```python
from build123d import *

# Parameters (mm, degrees)
F0_W     = 206
F0_H     = 56
F1_DEPTH = 3
F2_W     = 206
F2_H     = 56
F3_DEPTH = 10


with BuildPart() as f1:
    # F0 (on Top) → F1 (new body)
    with BuildSketch(Plane.XY):
        Rectangle(F0_W, F0_H)
    extrude(amount=F1_DEPTH)

    # F2 (on face) → F3 (join)
    with BuildSketch(Plane.XY.offset(3)):
        Rectangle(F2_W, F2_H)
        Polygon((100, -25), (-100, -25), (-100, 8.5), (100, -11.5), align=None, mode=Mode.SUBTRACT)
        Polygon((-100, 11.5), (-100, 25), (100, 25), (100, -8.5), align=None, mode=Mode.SUBTRACT)
    extrude(amount=F3_DEPTH)


solid = f1.part
```
Part model, mm, in its own coordinate system. A direction names the side the tool comes from. Round coordinates to 2 decimals unless told otherwise and drop trailing zeros. Loops run counter-clockwise (first coordinate to the right, second up) from the corner with the lowest first, then second, coordinate; pieces in that order, holes last.
Item 1: 3-axis set-ups, long thin cutter, end or side, ignore diameter. For faces 5 (the face through (103, 0, 6)), 6 (the face through (21, 12, 3)): which of +Z, -Z, +X, -X, +Y, -Y reach the whole face in a straight line?
Item 2: Drop a flat-ended pin along its axis: P1, Ø8, axis at x = -69.5, y = 13, coming from the +Z side. Give the stop position or say it passes through.
Item 3: Mould opens along Y. For faces 1 (the face through (1.4, 1.36, 7.93)), 2 (the face through (-1, -28, 6)), 3 (the face through (-1, 28, 6)), 4 (the face through (-8, 0, 13)) say: +Y half, -Y half, draft (parallel to the pull), parting line (faces both ways), or undercut.
Item 4: Drill centre lines: line 1 (X direction, y = -12, z = 10); line 2 (Y direction, x = 49, z = 4.25); line 3 (Y direction, x = -85, z = 8.5). Where is each one in solid material? Low to high.
Item 5: Cut at D-D, the plane y = 1. Give the cut face in (x, z).
Item 6: Cut at C-C, the plane y = -18. Give the cut face in (x, z), then the cut area to 3 significant figures.
Item 7: Cut at B-B, the plane x = -43. Give the cut face in (y, z), then the cut area to 3 significant figures.
Item 8: Cut at A-A, the plane z = 8.25. Give the cut face in (x, y), then the cut area to 3 significant figures.
A:
1. face 5: +Z, -Z, +X, +Y, -Y
1. face 6: +Z
2. P1: stops at z = 3
3. face 1: undercut
3. face 2: -Y half
3. face 3: +Y half
3. face 4: draft
4. line 1: x = -103 to -100, 100 to 103
4. line 2: y = -28 to -25, -6.4 to -3.4, 25 to 28
4. line 3: y = -28 to -25, 7 to 10, 25 to 28
5. outline: (-103, 0) - (103, 0) - (103, 13) - (100, 13) - (100, 3) - (5, 3) - (5, 13) - (-25, 13) - (-25, 3) - (-100, 3) - (-100, 13) - (-103, 13) - close
6. outline: (-103, 0) - (103, 0) - (103, 13) - (100, 13) - (100, 3) - (-100, 3) - (-100, 13) - (-103, 13) - close
6. area: 678 mm2
7. outline: (-28, 0) - (28, 0) - (28, 13) - (25, 13) - (25, 3) - (5.8, 3) - (5.8, 13) - (2.8, 13) - (2.8, 3) - (-25, 3) - (-25, 13) - (-28, 13) - close
7. area: 258 mm2
8. outline: (-103, -28) - (103, -28) - (103, 28) - (-103, 28) - close; hole (-100, -25) - (100, -25) - (100, -11.5) - (-100, 8.5) - close; hole (-100, 11.5) - (100, -8.5) - (100, 25) - (-100, 25) - close
8. area: 2,140 mm2
